Build history of the part. All positions in model axes, mm. Round coordinates to 2 decimals unless told otherwise and drop trailing zeros. Order: outer loops, then holes, each group sorted by start corner. A loop starts at its lowest first (then second) coordinate and runs counter-clockwise, first axis right, second up. Notation, with made-up numbers: M 38,13 L 88,13 A13 ccw 88,28 Z; hole C 31,47 d6. An arc over 180 degrees is marked long. One line per item, written item: value. Start each with the question number.
Item 1: Band-saw the part on D-D, the plane y = 3.5. Give the number of separate pieces and of enclosed holes in the cut face, then the cut area to 3 significant figures.
Item 2: Band-saw the part on A-A, the plane x = 172. Write the cut outline in (y, z).
Item 3: Pin check, flat tips, straight feed: pin 1 (4 mm diameter, centred on x = 110.49, z = -189.23, fed in from +Y); pin 2 (1 mm diameter, centred on x = 95, z = -107, fed in from -Y). Stop position of each tip, or through.
Item 4: Probe L1, parallel to X at y = 3, z = -100.5; L2, parallel to X at y = 2.25, z = -157; L3, parallel to Z at x = 42, y = 0.5. List the from-to ranges inside material, lowest first.
Item 5: Band-saw the part on C-C, the plane x = 80. Write the cut outline in (y, z).
Item 6: Two-plate mould, pull along X, no slides. Class faces 1 (the flat face through (199.98, 3.13, -200.07)), 2 (the flat face through (100, 3, -203.2)), 3 (the cylindrical face through (181.6, 3.22, -39.86)): +X half, -X half, draft (parallel to the pull), parting line (faces both ways), or undercut.
Item 7: Band-saw the part on B-B, the plane z = -54.5. Write the cut outline in (x, y), then the cut area to 3 significant figures.
```python
from build123d import *

# Parameters (mm, degrees)
BOSS_EXTRUDE1_DEPTH = 6.35
CUT_EXTRUDE1_DEPTH  = 288.438345563
SKETCH3_R           = 2.286
CUT_EXTRUDE2_DEPTH  = 288.438345563
BOSS_EXTRUDE2_DEPTH = 6.35
SKETCH5_R           = 4.826
BOSS_EXTRUDE3_DEPTH = 6.35
SKETCH6_R           = 2.286
CUT_EXTRUDE3_DEPTH  = 288.648691984


with BuildPart() as part:
    # Sketch1 → Boss-Extrude1 (new body)
    with BuildSketch(Plane(origin=(0, 0, 0), x_dir=(1, 0, 0), z_dir=(0, 1, 0))):
        Polygon((0, 196.85), (6.35, 203.2), (196.85, 203.2), (203.2, 196.85), (203.2, 6.35), (196.85, 0), (6.35, 0), (0, 6.35), align=None)
    extrude(amount=BOSS_EXTRUDE1_DEPTH)

    # Sketch2 → Cut-Extrude1 (cut, through all)
    with BuildSketch(Plane(origin=(0, 6.35, 0), x_dir=(1, 0, 0), z_dir=(0, 1, 0))):
        with BuildLine():
            Line((45.682614691, 185.42), (157.517385309, 185.42))
            ThreePointArc((157.517385309, 185.42), (163.384020341, 181.500039796), (162.00751337, 174.579871939))
            Line((162.00751337, 174.579871939), (106.090128061, 118.66248663))
            ThreePointArc((106.090128061, 118.66248663), (101.6, 116.802614691), (97.109871939, 118.66248663))
            Line((97.109871939, 118.66248663), (41.19248663, 174.579871939))
            ThreePointArc((41.19248663, 174.579871939), (39.815979659, 181.500039796), (45.682614691, 185.42))
        make_face()
        with BuildLine():
            Line((17.78, 157.517385309), (17.78, 45.682614691))
            ThreePointArc((17.78, 45.682614691), (21.699960204, 39.815979659), (28.620128061, 41.19248663))
            Line((28.620128061, 41.19248663), (84.53751337, 97.109871939))
            ThreePointArc((84.53751337, 97.109871939), (86.397385309, 101.6), (84.53751337, 106.090128061))
            Line((84.53751337, 106.090128061), (28.620128061, 162.00751337))
            ThreePointArc((28.620128061, 162.00751337), (21.699960204, 163.384020341), (17.78, 157.517385309))
        make_face()
        with BuildLine():
            Line((45.682614691, 17.78), (157.517385309, 17.78))
            ThreePointArc((157.517385309, 17.78), (163.384020341, 21.699960204), (162.00751337, 28.620128061))
            Line((162.00751337, 28.620128061), (106.090128061, 84.53751337))
            ThreePointArc((106.090128061, 84.53751337), (101.6, 86.397385309), (97.109871939, 84.53751337))
            Line((97.109871939, 84.53751337), (41.19248663, 28.620128061))
            ThreePointArc((41.19248663, 28.620128061), (39.815979659, 21.699960204), (45.682614691, 17.78))
        make_face()
        with BuildLine():
            Line((185.42, 157.517385309), (185.42, 45.682614691))
            ThreePointArc((185.42, 45.682614691), (181.500039796, 39.815979659), (174.579871939, 41.19248663))
            Line((174.579871939, 41.19248663), (118.66248663, 97.109871939))
            ThreePointArc((118.66248663, 97.109871939), (116.802614691, 101.6), (118.66248663, 106.090128061))
            Line((118.66248663, 106.090128061), (174.579871939, 162.00751337))
            ThreePointArc((174.579871939, 162.00751337), (181.500039796, 163.384020341), (185.42, 157.517385309))
        make_face()
    extrude(amount=-CUT_EXTRUDE1_DEPTH, mode=Mode.SUBTRACT)

    # Sketch3 → Cut-Extrude2 (cut, through all)
    with BuildSketch(Plane(origin=(0, 6.35, 0), x_dir=(1, 0, 0), z_dir=(0, 1, 0))):
        with Locations(Location((11.73734, 11.73734, 0), (0, 0, 270))):
            Circle(SKETCH3_R)
        with Locations(Location((191.46266, 11.73734, 0), (0, 0, 270))):
            Circle(SKETCH3_R)
        with Locations(Location((191.46266, 191.46266, 0), (0, 0, 270))):
            Circle(SKETCH3_R)
        with Locations(Location((11.73734, 191.46266, 0), (0, 0, 270))):
            Circle(SKETCH3_R)
    extrude(amount=-CUT_EXTRUDE2_DEPTH, mode=Mode.SUBTRACT)

    # Sketch4 → Boss-Extrude2 (add)
    with BuildSketch(Plane(origin=(0, 6.35, 0), x_dir=(1, 0, 0), z_dir=(0, 1, 0))):
        with BuildLine():
            Line((111.554726315, 185.42), (91.645273685, 185.42))
            ThreePointArc((91.645273685, 185.42), (94.961453031, 184.485298195), (97.301368182, 181.956363636))
            ThreePointArc((97.301368182, 181.956363636), (101.6, 179.324), (105.898631818, 181.956363636))
            ThreePointArc((105.898631818, 181.956363636), (108.238546969, 184.485298195), (111.554726315, 185.42))
        make_face()
    extrude(amount=-BOSS_EXTRUDE2_DEPTH)

    # Sketch5 → Boss-Extrude3 (add)
    with BuildSketch(Plane.XZ):
        with Locations(Location((101.6, -184.15, 0), (0, 0, 152.964308211))):
            Circle(SKETCH5_R)
    extrude(amount=BOSS_EXTRUDE3_DEPTH)

    # Sketch6 → Cut-Extrude3 (cut, through all)
    with BuildSketch(Plane.XZ.offset(6.35)):
        with Locations(Location((101.6, -184.15, 0), (0, 0, 270))):
            Circle(SKETCH6_R)
        with Locations(Location((92.71, -189.23, 0), (0, 0, 270))):
            Circle(SKETCH6_R)
        with Locations(Location((110.49, -189.23, 0), (0, 0, 270))):
            Circle(SKETCH6_R)
    extrude(amount=-CUT_EXTRUDE3_DEPTH, mode=Mode.SUBTRACT)


solid = part.part
```
Output:
1. separate pieces: 1
1. enclosed holes: 11
1. area: 21,300 mm²
2. outline: M 0,-203.2 L 6.35,-203.2 L 6.35,-159.43 L 0,-159.43 Z; M 0,-43.77 L 6.35,-43.77 L 6.35,0 L 0,0 Z
3. pin 1: passes through
3. pin 2: stops at y = 0
4. L1: x = 0 to 17.78, 86.3 to 116.9, 185.42 to 203.2
4. L2: x = 0 to 17.78, 33.63 to 58.77, 144.43 to 169.57, 185.42 to 203.2
4. L3: z = -203.2 to -184.24, -173.77 to -148.63, -54.57 to -29.43, -18.96 to 0
5. outline: M 0,-203.2 L 6.35,-203.2 L 6.35,-185.42 L 0,-185.42 Z; M 0,-135.77 L 6.35,-135.77 L 6.35,-110.63 L 0,-110.63 Z; M 0,-92.57 L 6.35,-92.57 L 6.35,-67.43 L 0,-67.43 Z; M 0,-17.78 L 6.35,-17.78 L 6.35,0 L 0,0 Z
6. face 1: +X half
6. face 2: draft
6. face 3: undercut
7. outline: M 0,0 L 17.78,0 L 17.78,6.35 L 0,6.35 Z; M 41.93,0 L 67.07,0 L 67.07,6.35 L 41.93,6.35 Z; M 136.13,0 L 161.27,0 L 161.27,6.35 L 136.13,6.35 Z; M 185.42,0 L 203.2,0 L 203.2,6.35 L 185.42,6.35 Z
7. area: 545 mm²
